Verification items for this drawing (mm, ordinates from the low corner). A direction names the side the tool comes from. Coordinates: 2 decimals unless noted, no trailing zeros. Write each loop counter-clockwise with the first axis right and the second up, starting at its lowest first coordinate (ties: lowest second). Pieces come first, ordered by that corner, then holes.
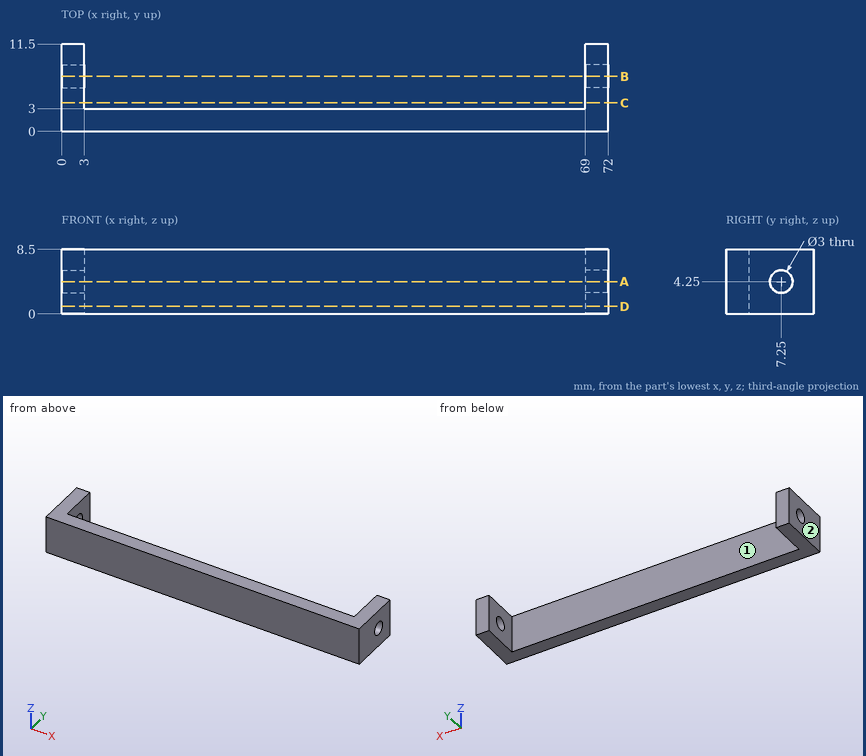
1. Sectioned sample at C-C, the plane y = 3.75. Record the boundary of the cut face in (x, z), and give its area (3 significant figures).
Computed values:
outline: (0, 0) - (3, 0) - (3, 8.5) - (0, 8.5) - close; (69, 0) - (72, 0) - (72, 8.5) - (69, 8.5) - close
area: 51.0 mm2
2. Sectioned sample at B-B, the plane y = 7.25. Record the boundary of the cut face in (x, z), and give its area (3 significant figures).
Computed values:
outline: (0, 0) - (3, 0) - (3, 2.75) - (0, 2.75) - close; (0, 5.75) - (3, 5.75) - (3, 8.5) - (0, 8.5) - close; (69, 0) - (72, 0) - (72, 2.75) - (69, 2.75) - close; (69, 5.75) - (72, 5.75) - (72, 8.5) - (69, 8.5) - close
area: 33.0 mm2
3. Gauge pin test, flat end, axial feed: pin 1 Ø4 at (x, z) = (30.5, 5.5) entering from +Y. Record the tip position at first contact, or that the pin passes through.
Computed values:
pin 1: stops at y = 3
4. Sectioned sample at D-D, the plane z = 1. Record the boundary of the cut face in (x, y).
Computed values:
outline: (0, 0) - (72, 0) - (72, 11.5) - (69, 11.5) - (69, 3) - (3, 3) - (3, 11.5) - (0, 11.5) - close
5. Thickness scan on line 1 along X through (y, z) = (6.25, 1.5); line 2 along Y through (x, z) = (70, 4.25); line 3 along Y through (x, z) = (56, 6). Record the ranges inside material, lowest first.
Computed values:
line 1: x = 0 to 3, 69 to 72
line 2: y = 0 to 5.75, 8.75 to 11.5
line 3: y = 0 to 3
6. Sectioned sample at A-A, the plane z = 4.25. Record the boundary of the cut face in (x, y).
Computed values:
outline: (0, 0) - (72, 0) - (72, 5.75) - (69, 5.75) - (69, 3) - (3, 3) - (3, 5.75) - (0, 5.75) - close; (0, 8.75) - (3, 8.75) - (3, 11.5) - (0, 11.5) - close; (69, 8.75) - (72, 8.75) - (72, 11.5) - (69, 11.5) - close
7. Access from +Z, -Z, +X, -X, +Y, -Y to the whole of each face (thin tool, end or side, straight path). Record for the marked faces 1 and 2.
Computed values:
face 1: +Z, -Z, +Y
face 2: +Z, -Z, -X, +Y, -Y
